Autodesk Inventor part; units mm, degrees
ref_plane "YZ Plane" through (0, 0, 0) normal (1, 0, 0) x (0, 1, 0)
ref_plane "XZ Plane" through (0, 0, 0) normal (0, 1, 0) x (-1, 0, 0)
ref_plane "XY Plane" through (0, 0, 0) normal (0, 0, 1) x (1, 0, 0)
sketch "構築線" plane through (0, 0, 0) normal (0, 0, 1) x (1, 0, 0)
  circle A0 centre (0, 0) radius 8.5
  circle A1 centre (0, 0) radius 2.8 construction
  circle A2 centre (0, 0) radius 5 construction
  line L0 (0, -8.6) -> (-25, -8.6) construction
  line L1 (0, -11.6) -> (-25, -11.6) construction
  circle A3 centre (-12.8148, 0.95) radius 10.05 construction
  circle A4 centre (-12.8148, 0.95) radius 12.55 construction
  circle A5 centre (0, 5) radius 0.8
  circle A6 centre (-4.3301, 2.5) radius 0.8
  circle A7 centre (-4.3301, -2.5) radius 0.8
  circle A8 centre (0, -5) radius 0.8
  circle A9 centre (4.3301, -2.5) radius 0.8
  circle A10 centre (4.3301, 2.5) radius 0.8
  line L2 (25, -8.6) -> (0, -8.6) construction
  circle A11 centre (12.8148, 0.95) radius 10.05 construction
  circle A12 centre (12.8148, 0.95) radius 12.55 construction
  line L3 (0, -11.6) -> (25, -11.6) construction
  line L4 (-22, -8.6) -> (0, -8.6)
  line L5 (0, 25) -> (0, -25)
  line L6 (0, -8.6) -> (22, -8.6)
  circle A13 centre (0, 0) radius 3
  circle A14 centre (0, 0) radius 1
  circle A15 centre (12.8148, 0.95) radius 1.05
  circle A16 centre (-12.8148, 0.95) radius 1.05
  circle A17 centre (12.8148, 0.95) radius 2.75
  circle A18 centre (-12.8148, 0.95) radius 2.75
  line L7 (-4.8008, 7.0144) -> (-17, 7.0144)
  line L8 (4.8008, 7.0144) -> (17, 7.0144)
  line L9 (-4.8008, 7.0144) -> (4.8008, 7.0144)
  line L10 (-17, 7.0144) -> (-22, 7.0144)
  line L11 (-22, 7.0144) -> (-22, -8.6)
  line L12 (22, -8.6) -> (22, 7.0144)
  line L13 (22, 7.0144) -> (17, 7.0144)
  dimension "d22" = 20.1
  dimension "d41" = 20.1
  dimension "d0" = 17
  dimension "d1" = 5.6
  dimension "d2" = 10
  dimension "d12" = 25
  dimension "d13" = 8.6
  dimension "d14" = 0
  dimension "d17" = 0
  dimension "d18" = 25
  dimension "d19" = 3
  dimension "d23" = 25.1
  dimension "d29" = 1.6
  dimension "d30" = 0
  dimension "d31" = 5
  dimension "d34" = 360
  dimension "d38" = 25
  dimension "d42" = 25.1
  dimension "d43" = 25
  dimension "d46" = 22
  dimension "d49" = 50
  dimension "d50" = 25
  dimension "d51" = 25
  dimension "d52" = 22
  dimension "d58" = 6
  dimension "d59" = 2
  dimension "d99" = 2.1
  dimension "d100" = 2.1
  dimension "d105" = 5.5
  dimension "d106" = 5.5
extrude "押し出し11" add sketch "構築線" along normal mid plane 4 contours A0 L5 A8 A13 A5 L9 | A0 L8 L13 L12 L6 L5 | L5 L4 L11 L10 L7 A0 | A0 L9 L5 A5 A13 A8 | A13 L5 A14 | L5 A14 A13 | A17 | A18
sketch "模様" plane through (0, 0, 2) normal (0, 0, 1) x (1, 0, 0)
  line L0 (-20, 5.5144) -> (-20, -7.1)
  line L1 (-20, -7.1) -> (20, -7.1) construction
  line L2 (-22, -8.6) -> (-22, 12.4) construction
  line L3 (-22, -8.6) -> (22, -8.6) construction
  line L4 (-20, 5.5144) -> (20, 5.5144) construction
  line L5 (20, 5.5144) -> (20, -7.1)
  line L6 (22, -8.6) -> (22, 12.4) construction
  line L7 (17, 7.0144) -> (-17, 7.0144) construction
  line L8 (-6.4685, 5.5144) -> (-20, 5.5144)
  line L9 (6.4685, 5.5144) -> (20, 5.5144)
  circle A0 centre (-12.8148, 0.95) radius 4 construction
  circle A1 centre (-12.8148, 0.95) radius 1.05
  line L10 (-12.8148, 0.95) -> (-12.8148, 4.95) construction
  line L11 (-12.8148, 0.95) -> (-16.8148, 0.95) construction
  line L12 (-12.8148, 4.95) -> (-15.1242, 0.95)
  line L13 (-15.1242, 0.95) -> (-12.8148, -3.05)
  line L14 (-12.8148, 4.95) -> (-10.5054, 0.95)
  line L15 (-10.5054, 0.95) -> (-12.8148, -3.05)
  circle A2 centre (0, 0) radius 1
  line L16 (-4.6733, -7.1) -> (-20, -7.1)
  line L17 (20, -7.1) -> (4.6733, -7.1)
  circle A3 centre (12.8148, 0.95) radius 4 construction
  circle A4 centre (0, 0) radius 8.5 construction
  arc A5 (-6.4685, 5.5144) -> (-4.6733, -7.1) centre (0, 0) ccw
  circle A6 centre (0, 0) radius 1
  circle A7 centre (12.8148, 0.95) radius 1.05
  arc A8 (4.6733, -7.1) -> (6.4685, 5.5144) centre (0, 0) ccw
  line L18 (12.8148, 0.95) -> (12.8148, 4.95) construction
  line L19 (12.8148, 0.95) -> (8.8148, 0.95) construction
  line L20 (12.8148, 4.95) -> (10.5054, 0.95)
  line L21 (10.5054, 0.95) -> (12.8148, -3.05)
  line L22 (12.8148, -3.05) -> (15.1242, 0.95)
  line L23 (15.1242, 0.95) -> (12.8148, 4.95)
  dimension "d166" = 17
  dimension "d135" = 2
  dimension "d136" = 1.5
  dimension "d137" = 2
  dimension "d138" = 1.5
  dimension "d139" = 8
  dimension "d140" = 60
  dimension "d141" = 60
  dimension "d142" = 60
  dimension "d143" = 60
  dimension "d145" = 8
  dimension "d167" = 60
  dimension "d168" = 60
  dimension "d169" = 60
sketch "スケッチ8" plane through (-22, 7.0144, 2) normal (0, 1, 0) x (1, 0, 0)
  line L0 (0.5, 0.5) -> (3.5, 0.5)
  line L1 (3.5, 0.5) -> (3.5, 3.5)
  line L2 (3.5, 3.5) -> (0.5, 3.5)
  line L3 (0.5, 3.5) -> (0.5, 0.5)
  line L4 (0.5, 0.5) -> (3.5, 3.5) construction
  line L5 (3.5, 0.5) -> (0.5, 3.5) construction
  line L6 (44, 0) -> (0, 0)
  line L7 (40.5, 0.5) -> (43.5, 0.5)
  line L8 (43.5, 0.5) -> (43.5, 3.5)
  line L9 (43.5, 3.5) -> (40.5, 3.5)
  line L10 (40.5, 3.5) -> (40.5, 0.5)
  line L11 (40.5, 0.5) -> (43.5, 3.5) construction
  line L12 (43.5, 0.5) -> (40.5, 3.5) construction
  point P0 (22, 2)
  point P1 (2, 2)
  point P2 (42, 2)
  dimension "d146" = 3
  dimension "d147" = 3
  dimension "d148" = 0.5
  dimension "d149" = 0.5
  dimension "d150" = 3
  dimension "d151" = 3
  dimension "d152" = 0.5
  dimension "d153" = 0.5
extrude "押し出し12" add sketch "スケッチ8" along normal blind 2
sketch "スケッチ9" plane through (-22, 9.0144, 2) normal (0, 1, 0) x (1, 0, 0)
  line L0 (4, 4) -> (0, 4)
  line L1 (0, 4) -> (0, 0)
  line L2 (0, 0) -> (4, 0)
  line L3 (4, 0) -> (4, 4)
  line L4 (4, 4) -> (0, 0) construction
  line L5 (0, 4) -> (4, 0) construction
  line L6 (0, 4) -> (0, 0)
  line L7 (44, 0) -> (0, 0)
  line L8 (40, 4) -> (44, 4)
  line L9 (44, 4) -> (44, 0)
  line L10 (44, 0) -> (40, 0)
  line L11 (40, 0) -> (40, 4)
  line L12 (40, 4) -> (44, 0) construction
  line L13 (44, 4) -> (40, 0) construction
  point P0 (22, 2)
  point P1 (2, 2)
  point P2 (42, 2)
  dimension "d156" = 4
  dimension "d157" = 4
  dimension "d158" = 2
  dimension "d159" = 2
  dimension "d160" = 4
  dimension "d161" = 4
  dimension "d162" = 2
  dimension "d163" = 2
extrude "押し出し13" add sketch "スケッチ9" along normal blind 2
extrude "押し出し16" cut sketch "模様" against normal blind 1 contours L8 A5 L16 L0 | L5 L17 A8 L9
sketch "固定穴" plane through (0, 0, -2) normal (0, 0, -1) x (-1, 0, 0)
  circle A0 centre (0, 0) radius 8.5
  line L0 (0, -8.6) -> (-25, -8.6) construction
  line L1 (25, -8.6) -> (0, -8.6) construction
  line L2 (0, 25) -> (0, -25)
  circle A1 centre (12.8148, 0.95) radius 2.75
  circle A2 centre (-12.8148, 0.95) radius 2.75
  circle A3 centre (0, 0) radius 1
  circle A4 centre (-12.8148, 0.95) radius 1.05
  circle A5 centre (12.8148, 0.95) radius 1.05
  circle A6 centre (0, 0) radius 2.8
  dimension "d180" = 17
  dimension "d183" = 25
  dimension "d195" = 25
  dimension "d200" = 50
  dimension "d208" = 5.5
  dimension "d209" = 5.5
  dimension "d216" = 5.6
extrude "押し出し19" cut sketch "固定穴" against normal blind 2 contours A1 | A2 | A4 | A5
extrude "押し出し20" cut sketch "固定穴" against normal blind 1 contours A0 L2 A6 | L2 A6 A0 | A6 L2 A3 | L2 A3 A6 | A3 L2 | L2 A3
extrude "押し出し21" cut sketch "固定穴" against normal blind 2.1 contours A6 L2 A3 | L2 A3 A6
sketch "ねじ穴+固定(基板)" plane through (-22, -8.6, 2) normal (0, -1, 0) x (1, 0, 0)
  circle A0 centre (38, -2) radius 1
  line L0 (44, -4) -> (44, 0)
  line L1 (44, -2) -> (0, -2) construction
  line L2 (0, -4) -> (0, 0)
  circle A1 centre (6, -2) radius 1
  line L3 (34.8, -3) -> (32.8, -3)
  line L4 (32.8, -3) -> (32.8, -1)
  line L5 (32.8, -1) -> (34.8, -1)
  line L6 (34.8, -1) -> (34.8, -3)
  line L7 (34.8, -3) -> (32.8, -1) construction
  line L8 (32.8, -3) -> (34.8, -1) construction
  line L9 (11.2, -1) -> (9.2, -1)
  line L10 (9.2, -1) -> (9.2, -3)
  line L11 (9.2, -3) -> (11.2, -3)
  line L12 (11.2, -3) -> (11.2, -1)
  line L13 (11.2, -1) -> (9.2, -3) construction
  line L14 (9.2, -1) -> (11.2, -3) construction
  point P0 (22, -2)
  point P1 (33.8, -2)
  point P2 (33.8, -2)
  point P3 (10.2, -2)
  point P4 (10.2, -2)
  dimension "d219" = 2
  dimension "d220" = 6
  dimension "d221" = 6
  dimension "d222" = 2
  dimension "d223" = 2
  dimension "d224" = 2
  dimension "d225" = 4.2
  dimension "d226" = 2
  dimension "d227" = 2
  dimension "d228" = 4.2
hole "ねじ穴(基板)" at (16, -8.6, 0) at (-16, -8.6, 0) direction (0, 1, 0) diameter 1.6 depth 3.5 tip angle 118
extrude "押し出し22" add sketch "ねじ穴+固定(基板)" along normal blind 1 contours L3 L4 L5 L6 | L12 L11 L10 L9
fillet "フィレット1" radius 0.5 4 edges at (12.8, -9.1, -1) (12.8, -9.1, 1) (10.8, -9.1, -1) (10.8, -9.1, 1)
fillet "フィレット2" radius 0.5 4 edges at (-12.8, -9.1, -1) (-12.8, -9.1, 1) (-10.8, -9.1, -1) (-10.8, -9.1, 1)
sketch "スケッチ12" plane through (-22, 11.0144, 2) normal (0, 1, 0) x (1, 0, 0)
  circle A0 centre (2, 2) radius 1
  line L0 (0, 0) -> (4, 0)
  line L1 (0, 4) -> (0, 0)
  circle A1 centre (42, 2) radius 1
  line L2 (44, 0) -> (44, 4)
  line L3 (40, 0) -> (44, 0)
  point P0 (22, 2)
  dimension "d240" = 2
  dimension "d241" = 2
  dimension "d242" = 2
  dimension "d243" = 2
  dimension "d244" = 2
  dimension "d245" = 2
hole "穴4" at (20, 11.0144, 0) at (-20, 11.0144, 0) direction (0, -1, 0) diameter 1.6 depth 3.5 tip angle 118
equation "\"d18\" = d12"
properties part number "mount2"
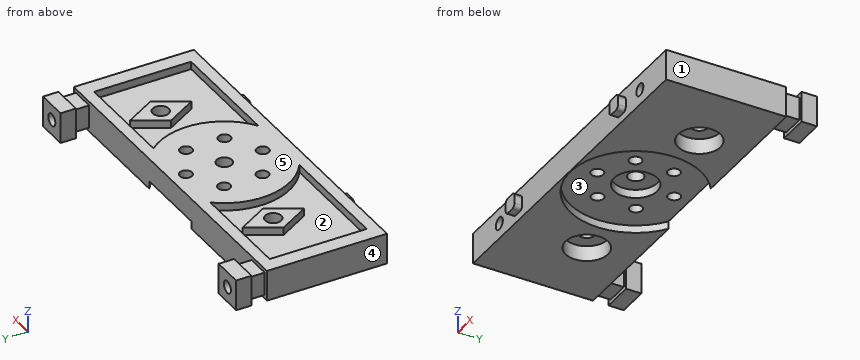
Read the model definition and answer for the solid it produces. Units are mm, in the model's axes. Face numbers are marked on the shaded views. A direction names the side the tool comes from. Round coordinates to 2 decimals unless told otherwise and drop trailing zeros. Write each loop counter-clockwise with the first axis right and the second up, starting at its lowest first coordinate (ties: lowest second). Pieces come first, ordered by that corner, then holes.
1. The part is cut by section A-A, the plane y = 8.5. Determine the outline of the cut face in (x, z).
2. Straight lines are drawn through the part: L1, parallel to X at y = 8.45, z = 0; L2, parallel to X at y = 9.25, z = -0.1; L3, parallel to Y at x = -16.5, z = 1.85. For each, find the intervals that lie inside material, in ascending order.
3. Determine the mould class of the marked faces 3, 4 and 5 for opening direction X: pulls with the +X half, pulls with the -X half, needs draft (parallel to the pull), parting line crosses it, or undercut.
4. The part is cut by section C-C, the plane x = -9. Determine the outline of the cut face in (y, z), then the cut area to 3 significant figures.
5. Which of the six approach directions +Z, -Z, +X, -X, +Y, -Y give full straight-line access (tool end or side, diameter ignored) to the marked faces 1 and 2?
6. The part is cut by section B-B, the plane x = 0. Determine the outline of the cut face in (y, z).
7. The part is cut by section D-D, the plane y = -7.75. Determine the outline of the cut face in (x, z), then the cut area to 3 significant figures.
8. Given pin 1 Ø1.1 at (x, y) = (12, -9) entering from +Z; pin 2 Ø3.5 at (x, y) = (0, 0) entering from -Z; pin 3 Ø0.5 at (x, z) = (-11.5, 1.5) entering from -Y; pin 4 Ø1 at (x, z) = (-16, 0) entering from +Y, each flat-ended and moving along its own axis, determine where each tip first touches the part or whether it passes through.
Values:
1. outline: (-21.5, -1.5) - (-18.5, -1.5) - (-18.5, 1.5) - (-21.5, 1.5) - close; (18.5, -1.5) - (21.5, -1.5) - (21.5, 1.5) - (18.5, 1.5) - close; hole circle Ø1.6 at (-20, 0); hole circle Ø1.6 at (20, 0)
2. L1: x = -21.5 to -20.8, -19.2 to -18.5, 18.5 to 19.2, 20.8 to 21.5
2. L2: x = -22 to -20.79, -19.21 to -18, 18 to 19.21, 20.79 to 22
2. L3: y = -8.6 to -7.1, 5.51 to 7.01
3. face 3: undercut
3. face 4: pulls with the -X half
3. face 5: needs draft
4. outline: (-8.6, -2) - (7.01, -2) - (7.01, 2) - (5.51, 2) - (5.51, 1) - (-7.1, 1) - (-7.1, 2) - (-8.6, 2) - close
4. area: 49.8 mm2
5. face 1: +Z, -Z, +X, +Y, -Y
5. face 2: +Z
6. outline: (-8.6, -2) - (-8.5, -2) - (-8.5, -1) - (-5.8, -1) - (-5.8, 2) - (-8.6, 2) - close; (-4.2, -1) - (-2.8, -1) - (-2.8, 0.1) - (-1, 0.1) - (-1, 2) - (-4.2, 2) - close; (1, 0.1) - (2.8, 0.1) - (2.8, -1) - (4.2, -1) - (4.2, 2) - (1, 2) - close; (5.8, -1) - (7.01, -1) - (7.01, 2) - (5.8, 2) - close
7. outline: (-22, -2) - (-3.49, -2) - (-3.49, -1) - (3.49, -1) - (3.49, -2) - (22, -2) - (22, 2) - (-22, 2) - close; hole circle Ø1.6 at (-16, 0); hole circle Ø1.6 at (16, 0)
7. area: 165 mm2
8. pin 1: stops at z = 2
8. pin 2: stops at z = 0.1
8. pin 3: stops at y = -8.6
8. pin 4: stops at y = 7.01
